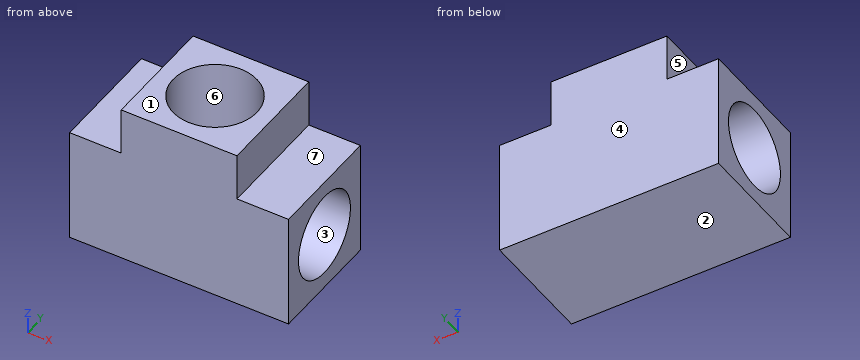
Autodesk Inventor part; units mm, degrees
ref_plane "YZ Plane" through (0, 0, 0) normal (1, 0, 0) x (0, 1, 0)
ref_plane "XZ Plane" through (0, 0, 0) normal (0, 1, 0) x (-1, 0, 0)
ref_plane "XY Plane" through (0, 0, 0) normal (0, 0, 1) x (1, 0, 0)
sketch "Sketch1" plane through (0, 0, 0) normal (0, 0, 1) x (1, 0, 0)
  line L0 (-13.4747, -7.1247) -> (13.4747, -7.1247)
  line L1 (13.4747, -7.1247) -> (13.4747, 7.1247)
  line L2 (13.4747, 7.1247) -> (-13.4747, 7.1247)
  line L3 (-13.4747, 7.1247) -> (-13.4747, -7.1247)
  line L4 (-13.4747, -7.1247) -> (13.4747, 7.1247) construction
  line L5 (13.4747, -7.1247) -> (-13.4747, 7.1247) construction
  line L6 (-7.1247, -7.1247) -> (7.1247, -7.1247)
  line L7 (7.1247, -7.1247) -> (7.1247, 7.1247)
  line L8 (7.1247, 7.1247) -> (-7.1247, 7.1247)
  line L9 (-7.1247, 7.1247) -> (-7.1247, -7.1247)
  line L10 (-7.1247, -7.1247) -> (7.1247, 7.1247) construction
  line L11 (7.1247, -7.1247) -> (-7.1247, 7.1247) construction
  point P0 (0, 0)
  dimension "d0" = 26.9494
  dimension "d1" = 14.2494
  dimension "d2" = 14.2494
extrude "Extrusion1" add sketch "Sketch1" along normal blind 5.8674 contours L9 L2 L7 L0
extrude "Extrusion2" add sketch "Sketch1" against normal blind 14.224
sketch "Sketch2" plane through (13.4747, -7.1247, 0) normal (1, 0, 0) x (0, 0, -1)
  line L0 (0, 0) -> (0, 14.2494) construction
  line L1 (0, 0) -> (14.224, 0) construction
  line L2 (14.224, 14.2494) -> (14.224, 0) construction
  line L3 (0, 14.2494) -> (14.224, 14.2494) construction
  circle A0 centre (7.0993, 7.1247) radius 7.1247 construction
  point P0 (0, 7.1247)
hole "Hole1" at (13.4747, 0, -7.0993) direction (-1, 0, 0) diameter 10.3124 end through all
sketch "Sketch3" plane through (0, 0, 5.8674) normal (0, 0, 1) x (1, 0, 0)
  point P0 (0, 0)
  point P1 (0, 0)
hole "Hole2" at (0, 0, 5.8674) direction (0, 0, -1) diameter 10.3124 end up to surface
properties part number "PPPP" material "Brass"
The listing builds one solid part. Answer for the finished solid, in the listing's coordinates (mm). Face numbers are marked on the shaded views. A direction names the side the tool comes from. Coordinates: 2 decimals unless noted, no trailing zeros. Loops run counter-clockwise (first coordinate to the right, second up) from the corner with the lowest first, then second, coordinate; pieces in that order, holes last. Notation, with made-up numbers: M 29,68.25 L 86,68.25 A11 cw 86,85.25 Z; hole C 75.5,17 d8. An arc over 180 degrees is marked long. Answer as a JSON object with one key per item and string values. Group by question number.
Item 1: Each of these flat-tipped pins is pushed along its axis until it touches: P1, Ø3, axis at y = -3, z = 4.5, coming from the +X side; P2, Ø1.9, axis at x = -10.5, y = -0.5, coming from the +Z side; P3, Ø1.8, axis at y = 1, z = 2, coming from the -X side. Where does it stop, or does it pass through?
Item 2: Section D-D (z = -2.25) is taken. Write down the section's boundary in (x, y).
Item 3: Which of the six approach directions +Z, -Z, +X, -X, +Y, -Y give full straight-line access (tool end or side, diameter ignored) to the marked faces 5, 6 and 7?
Item 4: Section A-A (y = 0) is taken. Write down the section's boundary in (x, z), and give its area (3 significant figures).
Item 5: Consider L1, parallel to Y at x = 0, z = -0.5; L2, parallel to Z at x = 5.25, y = 0. Determine where each line is inside the solid, lowest interval first.
Item 6: Determine the mould class of the marked faces 1, 2, 3 and 4 for opening direction Z: +Z half, -Z half, draft (parallel to the pull), parting line (faces both ways), or undercut.
Item 7: Section C-C (x = 0) is taken. Write down the section's boundary in (y, z).
Item 8: Section B-B (z = 2) is taken. Write down the section's boundary in (x, y).
Solved:
{
 "1": {"P1": "stops at x = 7.12", "P2": "stops at z = 0", "P3": "stops at x = -7.12"},
 "2": {"outline": "M -13.47,-7.12 L 13.47,-7.12 L 13.47,-1.75 L 4.85,-1.75 A5.16 cw -4.85,-1.75 L -13.47,-1.75 Z; M -13.47,1.75 L -4.85,1.75 A5.16 cw 4.85,1.75 L 13.47,1.75 L 13.47,7.12 L -13.47,7.12 Z"},
 "3": {"face 5": "+Z, -X, +Y, -Y", "face 6": "+Z", "face 7": "+Z, +X, +Y, -Y"},
 "4": {"outline": "M -13.47,-14.22 L 13.47,-14.22 L 13.47,-12.26 L -13.47,-12.26 Z; M -13.47,-1.94 L -5.16,-1.94 L -5.16,5.87 L -7.12,5.87 L -7.12,0 L -13.47,0 Z; M 5.16,-1.94 L 13.47,-1.94 L 13.47,0 L 7.12,0 L 7.12,5.87 L 5.16,5.87 Z", "area": "108 mm2"},
 "5": {"L1": "y = -7.12 to -5.16, 5.16 to 7.12", "L2": "z = -14.22 to -12.26, -1.94 to 5.87"},
 "6": {"face 1": "+Z half", "face 2": "-Z half", "face 3": "undercut", "face 4": "draft"},
 "7": {"outline": "M -7.12,-14.22 L 7.12,-14.22 L 7.12,5.87 L 5.16,5.87 L 5.16,-7.1 A5.16 cw -5.16,-7.1 L -5.16,5.87 L -7.12,5.87 Z"},
 "8": {"outline": "M -7.12,-7.12 L 7.12,-7.12 L 7.12,7.12 L -7.12,7.12 Z; hole C 0,0 d10.31"}
}
